Source: CAD feature listing. Evaluate the final solid. Frame: model axes, mm. A direction names the side the tool comes from. Give positions to 0.01 mm unless a question says otherwise; leave off trailing zeros. Order: outer loops, then holes, each group sorted by start corner. A loop starts at its lowest first (then second) coordinate and runs counter-clockwise, first axis right, second up. Notation, with made-up numbers: M 77.25,-29.5 L 95.25,-29.5 A13 ccw 95.25,-23.5 Z; hole C -14,45.25 d3. An arc over 180 degrees is marked long. Use CSV: the item, a comma, the result in double quotes. Start each with the question number.
1. Section query A-A, the plane x = 15. Return the cut outline in (y, z), plus the area to 3 significant figures.
2. Mould query, pull axis X, two halves, no side actions, for faces 1 (the flat face through (0, 7, 77)), 2 (the flat face through (91, 6, -10)), 3 (the flat face through (64, 6, -2)). Classes: released by +X, released by -X, zero draft, split by the parting line, or undercut.
3. Section query C-C, the plane y = -57. Return the cut outline in (x, z).
4. Section query B-B, the plane z = 73.5. Return the cut outline in (x, y).
5. Pin query (flat end, axial travel): P1, Ø2.5, axis at y = 2.5, z = 131, coming from the -X side; P2, Ø12, axis at x = 93, y = 0.5, coming from the -Z side; P3, Ø10, axis at x = 37, z = 203.5, coming from the -Y side; P4, Ø2, axis at x = 82, z = 166, coming from the -Y side. Return the tip coordinate at first contact, or that it passes through.
6. Reachability of faces 4 (the cylindrical face through (94.53, 8.03, -7.57)), 5 (the flat face through (66, 7, 77)), 6 (the flat face through (47, 2, 137)), 7 (the cylindrical face through (49.79, -3.01, 218.15)), 8 (the flat face through (5, 8, 159)) from +Z, -Z, +X, -X, +Y, -Y: full face, straight path, thin tool, end or side. Return the list, or none.
7. Section query D-D, the plane x = 40. Return the cut outline in (y, z).
8. Line query: line 1 along Y through (x, z) = (120, -4); line 2 along Z through (x, y) = (4, 1); line 3 along Y through (x, z) = (4, 224.75). Output: solid intervals per line, ascending. Write a range as [from, to].
Autodesk Inventor part; units mm, degrees
ref_plane "YZ Plane" through (0, 0, 0) normal (1, 0, 0) x (0, 1, 0)
ref_plane "XZ Plane" through (0, 0, 0) normal (0, 1, 0) x (-1, 0, 0)
ref_plane "XY Plane" through (0, 0, 0) normal (0, 0, 1) x (1, 0, 0)
sketch "草图5" plane through (0, 0, 0) normal (0, 1, 0) x (-1, 0, 0)
  line L0 (125, 235) -> (-125, 235)
  line L1 (-125, 235) -> (-125, -235)
  line L2 (-125, -235) -> (125, -235)
  line L3 (125, -235) -> (125, 235)
  line L4 (0, 3) -> (0, -5)
  line L5 (3.5058, 0) -> (-3.4421, 0)
  line L6 (25, 144) -> (-32, 144)
  line L7 (-32, 144) -> (-32, 87)
  line L8 (-32, 87) -> (25, 87)
  line L9 (25, 87) -> (25, 144)
  line L10 (25, 67) -> (-32, 67)
  line L11 (-32, 67) -> (-32, 10)
  line L12 (-32, 10) -> (25, 10)
  line L13 (25, 10) -> (25, 67)
  line L14 (25, -10) -> (-32, -10)
  line L15 (-32, -10) -> (-32, -67)
  line L16 (-32, -67) -> (25, -67)
  line L17 (25, -67) -> (25, -10)
  line L18 (25, -87) -> (-32, -87)
  line L19 (-32, -87) -> (-32, -144)
  line L20 (-32, -144) -> (25, -144)
  line L21 (25, -144) -> (25, -87)
  line L22 (-66, 100) -> (-95, 100)
  line L23 (-95, 100) -> (-95, 54)
  line L24 (-95, 54) -> (-66, 54)
  line L25 (-66, 54) -> (-66, 100)
  line L26 (-66, -54) -> (-95, -54)
  line L27 (-95, -54) -> (-95, -100)
  line L28 (-95, -100) -> (-66, -100)
  line L29 (-66, -100) -> (-66, -54)
  line L30 (100, 15) -> (70, 15)
  line L31 (70, 15) -> (70, -15)
  line L32 (70, -15) -> (100, -15)
  line L33 (100, -15) -> (100, 15)
  circle A0 centre (65, 182) radius 10
  circle A1 centre (65, -182) radius 10
  circle A2 centre (65, 182) radius 15
  circle A3 centre (80, 182) radius 1.5
  circle A4 centre (57.5, 194.9904) radius 1.5
  circle A5 centre (57.5, 169.0096) radius 1.5
  line L34 (125, 235) -> (0, 235)
  line L35 (0, 235) -> (0, 0)
  line L36 (0, 0) -> (125, 0)
  line L37 (125, 0) -> (125, 235)
  line L38 (-125, 235) -> (0, 235)
  line L39 (0, 235) -> (0, 0)
  line L40 (0, 0) -> (-125, 0)
  line L41 (-125, 0) -> (-125, 235)
  line L42 (-125, -235) -> (0, -235)
  line L43 (0, -235) -> (0, 0)
  line L44 (0, 0) -> (-125, 0)
  line L45 (-125, 0) -> (-125, -235)
  line L46 (125, -235) -> (0, -235)
  line L47 (0, -235) -> (0, 0)
  line L48 (0, 0) -> (125, 0)
  line L49 (125, 0) -> (125, -235)
  circle A6 centre (65, -182) radius 15
  circle A7 centre (80, -182) radius 1.5
  circle A8 centre (57.5, -169.0096) radius 1.5
  circle A9 centre (57.5, -194.9904) radius 1.5
  point P0 (0, 67)
  point P1 (0, 87)
  point P2 (0, 144)
  point P3 (0, 10)
  dimension "d142" = 30
  dimension "d145" = 30
  dimension "d111" = 470
  dimension "d112" = 250
  dimension "d113" = 57
  dimension "d114" = 57
  dimension "d115" = 57
  dimension "d116" = 57
  dimension "d117" = 57
  dimension "d118" = 57
  dimension "d119" = 57
  dimension "d120" = 57
  dimension "d121" = 91
  dimension "d122" = 20
  dimension "d123" = 20
  dimension "d124" = 20
  dimension "d125" = 93
  dimension "d126" = 29
  dimension "d127" = 46
  dimension "d128" = 46
  dimension "d129" = 135
  dimension "d130" = 108
  dimension "d131" = 30
  dimension "d132" = 30
  dimension "d133" = 30
  dimension "d134" = 25
  dimension "d135" = 220
  dimension "d136" = 20
  dimension "d137" = 53
  dimension "d138" = 60
  dimension "d139" = 20
  dimension "d140" = 53
  dimension "d141" = 60
  dimension "d143" = 3
  dimension "d144" = 360
  dimension "d146" = 3
  dimension "d147" = 360
extrude "拉伸5" add sketch "草图5" along normal blind 10 contours L35 L6 L7 L8 L10 L11 L12 L4 L5 L40 L1 L0
sketch "草图6" plane through (0, 0, 0) normal (0, -1, 0) x (1, 0, 0)
  line L0 (125, 0) -> (0, 0)
  line L1 (0, 144) -> (0, 235)
  line L2 (47, 0) -> (0, 0)
  line L3 (0, 0) -> (0, 159)
  line L4 (0, 159) -> (47, 159)
  line L5 (47, 159) -> (47, 0)
  line L6 (32, 87) -> (32, 144)
  line L7 (32, 144) -> (0, 144)
  line L8 (111, 115) -> (47, 115)
  line L9 (47, 115) -> (47, 39)
  line L10 (47, 39) -> (111, 39)
  line L11 (111, 39) -> (111, 115)
  line L12 (95, 54) -> (95, 100)
  line L13 (95, 100) -> (66, 100)
  line L14 (66, 54) -> (95, 54)
  line L15 (66, 100) -> (66, 54)
  dimension "d150" = 15
  dimension "d151" = 15
  dimension "d152" = 16
  dimension "d153" = 15
  dimension "d154" = 15
  dimension "d155" = 19
extrude "拉伸6" cut sketch "草图6" against normal blind 5 contours L0 L3 L1 L4 L5 | L5 L8 L11 L10 | L14 L15 L13 L12
sketch "草图7" plane through (0, 10, 0) normal (0, 1, 0) x (1, 0, 0)
  line L0 (0, -144) -> (0, -159)
  line L1 (0, -235) -> (125, -235)
  line L2 (0, -159) -> (10, -159)
  line L3 (10, -159) -> (10, -235)
  line L4 (10, -235) -> (0, -235)
  line L5 (0, -235) -> (0, -159)
  point P0 (0, 0)
  dimension "d158" = 10
extrude "拉伸7" cut sketch "草图7" against normal blind 5
sketch "草图8" plane through (0, 5, 0) normal (0, 1, 0) x (1, 0, 0)
  circle A0 centre (4, -205) radius 2.1
  circle A1 centre (4, -179) radius 2.1
  line L0 (0, -235) -> (0, -159)
  line L1 (10, -235) -> (0, -235)
  line L2 (32, -144) -> (0, -144)
  line L3 (0, -159) -> (10, -159)
  point P0 (0, 0)
  dimension "d161" = 4.2
  dimension "d162" = 4.2
  dimension "d163" = 4
  dimension "d164" = 4
  dimension "d165" = 30
  dimension "d169" = 20
extrude "拉伸8" cut sketch "草图8" against normal blind 5
sketch "草图9" plane through (0, 0, 0) normal (0, -1, 0) x (1, 0, 0)
  line L0 (125, 0) -> (0, 0)
  line L1 (0, 235) -> (125, 235)
  line L2 (125, 0) -> (111, 0)
  line L3 (111, 0) -> (111, 235)
  line L4 (111, 235) -> (125, 235)
  line L5 (125, 235) -> (125, 0)
  line L6 (0, 159) -> (0, 235)
  line L7 (125, 235) -> (125, 0)
  line L8 (0, 235) -> (125, 235)
  line L9 (125, 235) -> (125, 221)
  line L10 (125, 221) -> (0, 221)
  line L11 (0, 221) -> (0, 235)
  point P0 (0, 221)
  point P1 (111, 221)
  dimension "d170" = 14
  dimension "d171" = 14
extrude "拉伸9" add sketch "草图9" along normal blind 70
sketch "草图10" plane through (10, 10, 235) normal (0, 0, 1) x (1, 0, 0)
  line L0 (0, -5) -> (-10, -5)
  line L1 (-10, -80) -> (-10, -5)
  line L2 (0, -5) -> (-10, -5)
  line L3 (-10, -5) -> (-10, -80)
  line L4 (-10, -80) -> (0, -80)
  line L5 (0, -80) -> (0, -5)
  point P0 (-10, -10)
extrude "拉伸10" cut sketch "草图10" against normal blind 7
sketch "草图11" plane through (10, 10, 228) normal (0, 0, 1) x (1, 0, 0)
  circle A0 centre (-6, -30) radius 2.1
  circle A1 centre (-6, -60) radius 2.1
  line L0 (-10, -80) -> (-10, -5)
  line L1 (0, -80) -> (-10, -80)
  line L2 (0, 0) -> (115, 0)
  point P0 (-10, -10)
  dimension "d176" = 4.2
  dimension "d177" = 4.2
  dimension "d178" = 4
  dimension "d179" = 4
  dimension "d180" = 20
  dimension "d181" = 30
extrude "拉伸11" cut sketch "草图11" against normal blind 7
fillet "圆角2" radius 10 4 edges at (111, 0, 168) (111, 0, 19.5) (111, -35, 221) (55.5, 0, 221)
sketch "草图12" plane through (0, 0, 0) normal (0, -1, 0) x (1, 0, 0)
  circle A0 centre (65, 175) radius 10
  line L0 (125, 0) -> (125, 235)
  line L1 (125, 235) -> (10, 235)
  point P0 (0, 0)
  point P1 (125, 230)
  point P2 (120, 235)
  dimension "d186" = 20
  dimension "d187" = 60
  dimension "d188" = 60
extrude "拉伸12" add sketch "草图12" along normal blind 70
fillet "圆角3" radius 10 1 edges at (55, 0, 175)
sketch "草图14" plane through (125, 10, 235) normal (1, 0, 0) x (0, 0, -1)
  line L0 (235, -80) -> (235, 0)
  line L1 (235, 0) -> (245, 0)
  line L2 (245, 0) -> (245, -80)
  line L3 (245, -80) -> (235, -80)
  line L4 (235, -80) -> (235, 0)
  line L5 (0, 0) -> (235, 0)
  circle A0 centre (239, -60) radius 2.1
  circle A1 centre (239, -30) radius 2.1
  point P0 (235, -10)
  dimension "d192" = 10
  dimension "d193" = 80
  dimension "d196" = 4.2
  dimension "d197" = 4.2
  dimension "d198" = 6
  dimension "d199" = 6
  dimension "d200" = 20
  dimension "d201" = 30
extrude "拉伸14" add sketch "草图14" against normal blind 7
sketch "草图15" plane through (0, 10, 0) normal (0, 1, 0) x (1, 0, 0)
  line L0 (118, 0) -> (0, 0)
  circle A0 centre (95, 4) radius 2.1
  circle A1 centre (62, 4) radius 2.1
  line L1 (125, -235) -> (125, 10)
  line L2 (118, 0) -> (32, 0)
  line L3 (32, 0) -> (32, 10)
  line L4 (32, 10) -> (118, 10)
  line L5 (118, 10) -> (118, 0)
  line L6 (32, -10) -> (32, -67)
  line L7 (125, 10) -> (118, 10)
  point P0 (32, 0)
  dimension "d205" = 4.2
  dimension "d206" = 4.2
  dimension "d209" = 30
  dimension "d212" = 6
  dimension "d213" = 6
  dimension "d214" = 30
extrude "拉伸15" add sketch "草图15" against normal blind 5
sketch "草图16" plane through (0, 10, 0) normal (0, 1, 0) x (1, 0, 0)
  circle A0 centre (95, 4) radius 2.1
  circle A1 centre (95, 4) radius 3.6
  circle A2 centre (62, 4) radius 2.1
  circle A3 centre (62, 4) radius 3.6
  point P0 (0, 0)
  dimension "d217" = 7.2
  dimension "d218" = 7.2
extrude "拉伸16" cut sketch "草图16" against normal blind 4
sketch "草图17" plane through (125, -70, 235) normal (1, 0, 0) x (0, 0, -1)
  circle A0 centre (239, 50) radius 2.1
  circle A1 centre (239, 50) radius 3.6
  circle A2 centre (239, 20) radius 2.1
  circle A3 centre (239, 20) radius 3.6
  point P0 (235, 70)
  dimension "d221" = 7.2
  dimension "d222" = 7.2
extrude "拉伸17" cut sketch "草图17" against normal blind 4
fillet "圆角4" radius 5 3 edges at (125, 10, 112.5) (67.5, 10, 235) (125, -30, 235)
sketch "草图18" plane through (0, 10, 0) normal (0, 1, 0) x (1, 0, 0)
  line L0 (0, 0) -> (0, -10)
  line L1 (32, 10) -> (118, 10)
  line L2 (0, 0) -> (32, 0)
  line L3 (32, 0) -> (32, 10)
  line L4 (32, 10) -> (0, 10)
  line L5 (0, 10) -> (0, 0)
extrude "拉伸18" add sketch "草图18" against normal blind 5
sketch "草图20" plane through (0, -70, 0) normal (0, -1, 0) x (1, 0, 0)
  circle A0 centre (65, 175) radius 10
  circle A1 centre (65, 175) radius 10
  line L0 (111, 211) -> (111, 0)
  line L1 (0, 221) -> (101, 221)
  point P0 (0, 0)
  dimension "d228" = 46
  dimension "d229" = 46
properties part number "top_3"
Result set:
1,outline,"M -70,221 L -10,221 A10 cw 0,211 L 0,159 L 5,159 L 5,144 L 10,144 L 10,230 A5 ccw 5,235 L -70,235 Z; M 5,-10 L 10,-10 L 10,10 L 5,10 Z; M 5,67 L 10,67 L 10,87 L 5,87 Z"
1,area,"2,030 mm2"
2,face 1,"released by -X"
2,face 2,"zero draft"
2,face 3,"undercut"
3,outline,"M 0,221 L 101,221 A10 cw 111,211 L 111,0 L 118,0 L 118,-10 L 125,-10 L 125,230 A5 ccw 120,235 L 10,235 L 10,228 L 0,228 Z; C 65,175 d20"
4,outline,"M 0,5 L 66,5 L 66,10 L 0,10 Z; M 95,5 L 111,5 L 111,-70 L 125,-70 L 125,5 A5 ccw 120,10 L 95,10 Z"
5,P1,"x = 47"
5,P2,"z = -10"
5,P3,"y = 0"
5,P4,"y = -0.16"
6,face 4,"+Y"
6,face 5,"+Y, -Y"
6,face 6,"-Z, -X, -Y"
6,face 7,"-X, -Y"
6,face 8,"+Z, -X, +Y"
7,outline,"M -70,221 L -10,221 A10 cw 0,211 L 0,159 L 5,159 L 5,-10 L 10,-10 L 10,230 A5 ccw 5,235 L -70,235 Z"
8,line 1,"[-70, -52.1], [-47.9, -22.1], [-17.9, 10]"
8,line 2,"[159, 176.9], [181.1, 202.9], [207.1, 228]"
8,line 3,"[-70, -52.1], [-47.9, -22.1], [-17.9, 5]"
